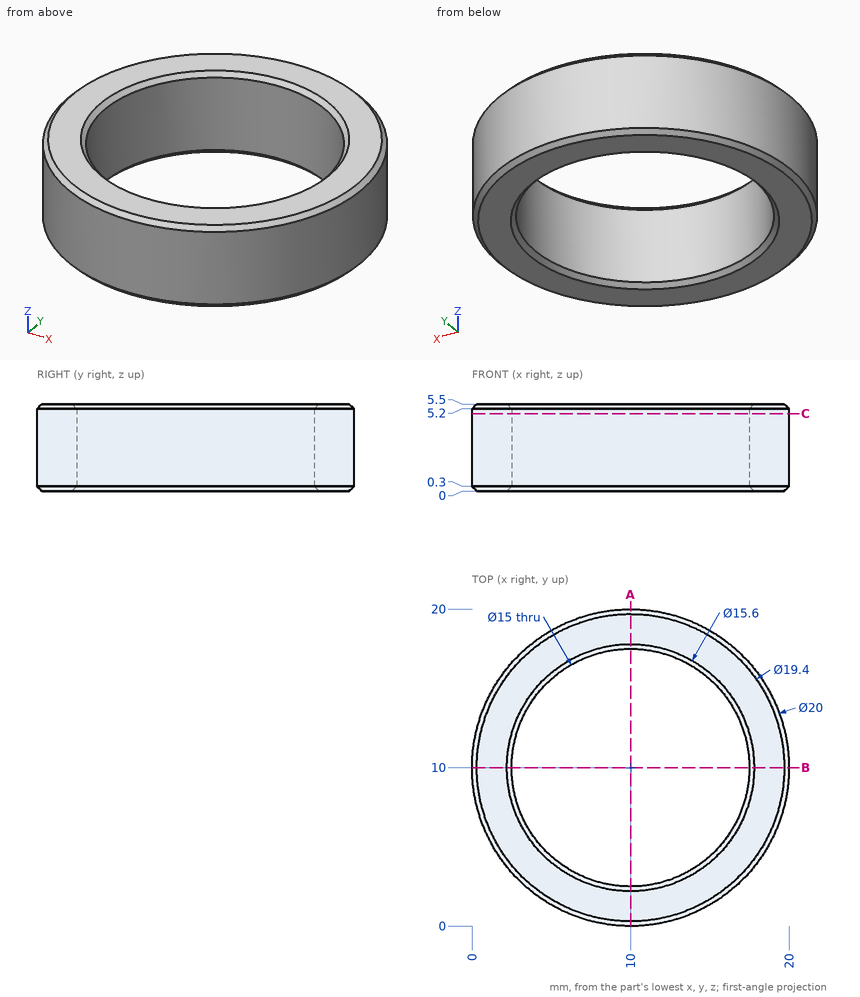
Input: dimensioned drawing with shaded views. Units: mm. Origin: part minimum x, y, z. Round coordinates to 2 decimals unless told otherwise and drop trailing zeros. Order: outer loops, then holes, each group sorted by start corner. A loop starts at its lowest first (then second) coordinate and runs counter-clockwise, first axis right, second up. Notation, with made-up numbers: (10.5, 17) -> (17.5, 17) arc R28 ccw to (17.5, 49) -> close; hole circle Ø10 at (14, 45.25). An arc over 180 degrees is marked (long way). Put each result on its own line as item: value. Start each with the question number.
Q1. First-contact query: pin 1 (1 mm diameter, centred on y = 6, z = 1, fed in from +X); pin 2 (1 mm diameter, centred on y = 17, z = 3.5, fed in from +X); pin 3 (9 mm diameter, centred on x = 10, y = 10, fed in from +Z); pin 4 (1.5 mm diameter, centred on x = 11, z = 4, fed in from +Y). Flat tips, straight axial feed; report the tip coordinate or a pass-through.
Q2. Line query: probe 1 along Y at (x, z) = (10, 3.05); probe 2 along Y at (x, z) = (11.25, 3); probe 3 along X at (y, z) = (7.25, 5.25). Output: solid intervals per line, ascending.
Q3. Section C-C on z = 4.9. Return the cut outline in (x, y), and give its area (3 significant figures).
Q4. Section A-A on x = 10. Return the cut outline in (y, z).
Ans:
1. pin 1: stops at x = 19.37
1. pin 2: stops at x = 17.6
1. pin 3: passes through
1. pin 4: stops at y = 20
2. probe 1: y = 0 to 2.5, 17.5 to 20
2. probe 2: y = 0.08 to 2.6, 17.4 to 19.92
2. probe 3: x = 0.44 to 2.97, 17.03 to 19.56
3. outline: circle Ø20 at (10, 10); hole circle Ø15 at (10, 10)
3. area: 137 mm2
4. outline: (0, 0.3) -> (0.3, 0) -> (2.2, 0) -> (2.5, 0.3) -> (2.5, 5.2) -> (2.2, 5.5) -> (0.3, 5.5) -> (0, 5.2) -> close; (17.5, 0.3) -> (17.8, 0) -> (19.7, 0) -> (20, 0.3) -> (20, 5.2) -> (19.7, 5.5) -> (17.8, 5.5) -> (17.5, 5.2) -> close
